Geometry: final body of the model. Coordinates: model frame, mm. A direction names the side the tool comes from. Coordinates: 2 decimals unless noted, no trailing zeros. Write each loop counter-clockwise with the first axis right and the second up, starting at its lowest first coordinate (ties: lowest second). Pieces come first, ordered by that corner, then holes. Notation, with made-up numbers: (77, 51) -> (98, 51) arc R18 ccw to (98, 80) -> close; hole circle Ø3 at (12, -17.75). An arc over 180 degrees is marked (long way). Answer as a JSON object with one key per item and string values. Group by question number.
```python
from build123d import *

# Parameters (mm, degrees)
BOSS_EXTRUDE1_START                    = 1.27
BOSS_EXTRUDE1_DEPTH                    = 20.586143
F_4_40_TAPPED_HOLE1_D                  = 2.2606
F_1_8_0_125_DIAMETER_HOLE1_D           = 3.175
F_1_8_0_125_DIAMETER_HOLE1_CSINK_D     = 4.445
F_1_8_0_125_DIAMETER_HOLE1_CSINK_ANGLE = 100
CUT_EXTRUDE1_DEPTH                     = 8.255
CUT_EXTRUDE2_DEPTH                     = 21.586143296


with BuildPart() as part:
    # Sketch1 → Boss-Extrude1 (new body)
    with BuildSketch(Plane.XY.offset(BOSS_EXTRUDE1_START)):
        Polygon((8.016705611, -68.938838733), (7.029985744, -71.956620849), (0.99442151, -69.983181117), (0.007701644, -73.000963234), (-12.063426824, -69.054083768), (-14.036866557, -75.089648002), (11.365311403, -83.395361493), (15.229120806, -71.578294343), (12.021207594, -66.907776482), (9.003425477, -65.921056616), align=None)
    extrude(amount=BOSS_EXTRUDE1_DEPTH)

    # #4-40 Tapped Hole1 (through all)
    with Locations(Plane.XY.offset(21.856143296)):
        with Locations((-9.766799747, -73.145417099)):
            Hole(F_4_40_TAPPED_HOLE1_D / 2)

    # 1/8 (0.125) Diameter Hole1 (through all)
    with Locations(Plane.XY.offset(21.856143296)):
        with Locations((8.997580837, -79.280779556)):
            CounterSinkHole(F_1_8_0_125_DIAMETER_HOLE1_D / 2, F_1_8_0_125_DIAMETER_HOLE1_CSINK_D / 2, counter_sink_angle=F_1_8_0_125_DIAMETER_HOLE1_CSINK_ANGLE)

    # Sketch6 → Cut-Extrude1 (cut)
    with BuildSketch(Plane(origin=(-23.536376178, -71.983607041, 0), x_dir=(0.950482557, -0.310777911, 0), z_dir=(-0.310777911, -0.950482557, 0))):
        with BuildLine():
            Line((36.719966444, 13.150571648), (26.559966444, 13.150571648))
            ThreePointArc((26.559966444, 13.150571648), (24.972466444, 11.563071648), (26.559966444, 9.975571648))
            Line((26.559966444, 9.975571648), (36.719966444, 9.975571648))
            ThreePointArc((36.719966444, 9.975571648), (38.307466444, 11.563071648), (36.719966444, 13.150571648))
        make_face()
    extrude(amount=-CUT_EXTRUDE1_DEPTH, mode=Mode.SUBTRACT)

    # Sketch8 → Cut-Extrude2 (cut, through all)
    with BuildSketch(Plane.XY.offset(21.856143296)):
        with BuildLine():
            Line((-5.462102823, -72.94952157), (-2.685743275, -73.857303847))
            ThreePointArc((-2.685743275, -73.857303847), (-0.165929608, -73.663685373), (1.478938787, -71.744999106))
            ThreePointArc((1.478938787, -71.744999106), (1.632876898, -70.97000506), (1.598291814, -70.180627719))
            Line((1.598291814, -70.180627719), (0.99442151, -69.983181117))
            Line((0.99442151, -69.983181117), (0.007701644, -73.000963234))
            Line((0.007701644, -73.000963234), (-7.667023508, -70.491569419))
            ThreePointArc((-7.667023508, -70.491569419), (-6.893866312, -72.015948853), (-5.462102823, -72.94952157))
        make_face()
        with BuildLine():
            ThreePointArc((1.598291814, -70.180627719), (1.632876898, -70.97000506), (1.478938787, -71.744999106))
            Line((1.478938787, -71.744999106), (1.952564323, -70.29646369))
            Line((1.952564323, -70.29646369), (1.598291814, -70.180627719))
        make_face()
    extrude(amount=-CUT_EXTRUDE2_DEPTH, mode=Mode.SUBTRACT)


solid = part.part
```
Item 1: Section A-A on z = 3.25. Output: boundary loops of the cut face in (x, y) (1 decimal).
Item 2: Section B-B on x = -10. Output: boundary loops of the cut face in (y, z).
Item 3: Set-up query: faces 4 (the flat face through (-4.09, -73.4, 11.71)), 5 (the flat face through (-1.514, -79.184, 11.419)), 6 (the cylindrical face through (1.465, -75.876, 11.598)). Return all of +Z, -Z, +X, -X, +Y, -Y with unobstructed straight access to the full face (end or side cutting, diameter ignored); none if empty.
Item 4: Mould query, pull axis X, two halves, no side actions, for faces 1 (the flat face through (-13.036, -72.03, 11.419)), 2 (the flat face through (13.27, -77.57, 9.13)), 3 (the cylindrical face through (9.204, -77.707, 5.562)). Classes: +X half, -X half, draft (parallel to the pull), parting line (faces both ways), or undercut.
Item 5: Contact query for flat-ended pins moving along their axis: pin 1 (3 mm diameter, centred on x = 9, y = -79.28, fed in from -Z); pin 2 (1 mm diameter, centred on x = -6.5, z = 6.5, fed in from -Y); pin 3 (12 mm diameter, centred on x = -6, z = 5.5, fed in from +Y); pin 4 (5 mm diameter, centred on x = -2.5, z = 6, fed in from +Y). Output: stop coordinate, or through.
Item 6: Ray query, L1, parallel to Z at x = 6.25, y = -75.5; L2, parallel to Z at x = 10, y = -78; L3, parallel to Y at x = 0.75, z = 9.75. Return the intervals inside material, ascending. Write a range as [from, to].
Item 7: Section D-D on z = 10.5. Output: boundary loops of the cut face in (x, y) (3 decimals), then the cut area to 3 significant figures.
Item 8: Section C-C on y = -79.75. Give the number of separate pieces and of enclosed holes in the cut face, then the cut area to 3 significant figures.
Answer sheet:
{
 "1": {"outline": "(-14, -75.1) -> (11.4, -83.4) -> (15.2, -71.6) -> (12, -66.9) -> (9, -65.9) -> (7, -72) -> (2, -70.3) -> (1.5, -71.7) arc R3.3 cw to (-2.7, -73.9) -> (-5.5, -72.9) arc R3.3 cw to (-7.7, -70.5) -> (-12.1, -69.1) -> close; hole circle Ø2.3 at (-9.8, -73.1); hole circle Ø3.2 at (9, -79.3)"},
 "2": {"outline": "(-76.41, 1.27) -> (-74.25, 1.27) -> (-74.25, 21.86) -> (-76.41, 21.86) -> close; (-72.04, 1.27) -> (-69.73, 1.27) -> (-69.73, 21.86) -> (-72.04, 21.86) -> close"},
 "3": {"face 4": "+Z, -Z, +Y", "face 5": "+Z, -Z, -X, -Y", "face 6": "-Y"},
 "4": {"face 1": "-X half", "face 2": "+X half", "face 3": "undercut"},
 "5": {"pin 1": "passes through", "pin 2": "stops at y = -77.72", "pin 3": "stops at y = -69.07", "pin 4": "stops at y = -73.1"},
 "6": {"L1": "z = [1.27, 9.98], [13.15, 21.86]", "L2": "z = [1.27, 9.98], [13.15, 21.36]", "L3": "y = [-79.92, -72.98]"},
 "7": {"outline": "(-14.037, -75.09) -> (0.588, -79.871) -> (3.153, -72.025) -> (13.931, -75.549) -> (15.229, -71.578) -> (12.021, -66.908) -> (9.003, -65.921) -> (7.03, -71.957) -> (1.953, -70.296) -> (1.479, -71.745) arc R3.302 cw to (-2.686, -73.857) -> (-5.462, -72.95) arc R3.302 cw to (-7.667, -70.492) -> (-12.063, -69.054) -> close; hole circle Ø2.261 at (-9.767, -73.145)", "area": "143 mm^2"},
 "8": {"separate pieces": "4", "enclosed holes": "0", "area": "163 mm^2"}
}
